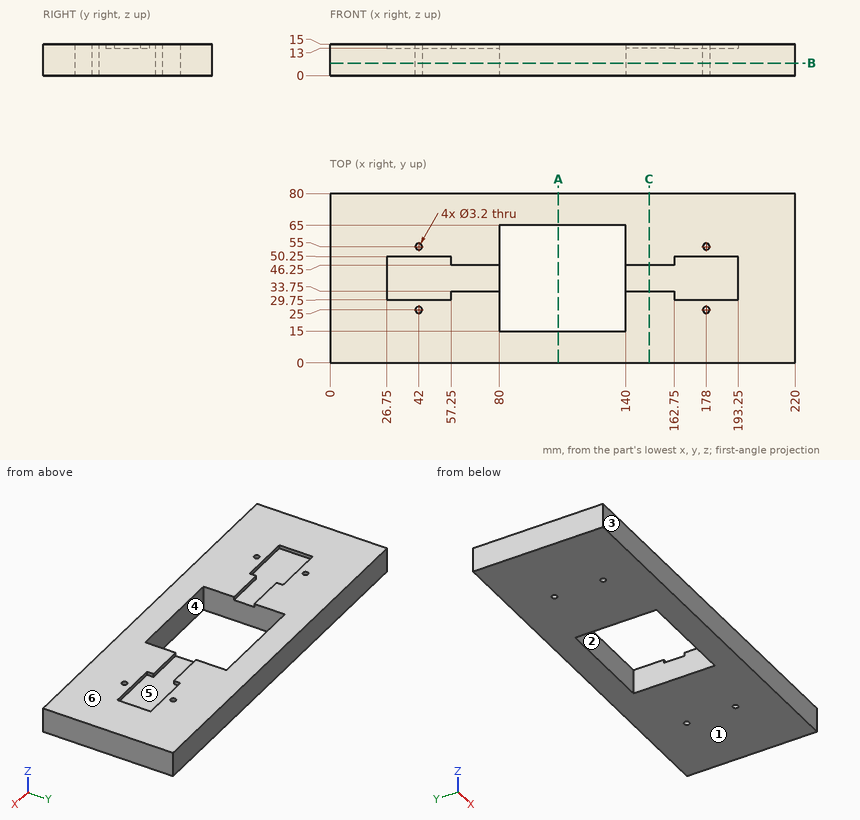
Part print with two shaded views. Sizes in mm from the minimum x, y, z corner. A direction names the side the tool comes from. Coordinates: 2 decimals unless noted, no trailing zeros. Write each loop counter-clockwise with the first axis right and the second up, starting at its lowest first coordinate (ties: lowest second). Pieces come first, ordered by that corner, then holes. Notation, with made-up numbers: M -29,-35.75 L 24,-35.75 A36 ccw 24,3.25 Z; hole C 45.25,30.25 d9. An arc over 180 degrees is marked long. Return JSON: item names as keys, results as strings.
Item 1: Which spindle directions (+Z, -Z, +X, -X, +Y, -Y) get a long thin tool onto all of the face, cutting with end or side? Do the marked faces 1 and 2. Say none if no direction does.
Findings below:
{"face 1": "-Z, +X, -X, +Y, -Y", "face 2": "+Z, -Z"}
Item 2: Slice it at B-B, the plane z = 6. Write the cut outline in (x, y).
Findings below:
{"outline": "M 0,0 L 220,0 L 220,80 L 0,80 Z; hole C 42,25 d3.2; hole C 42,55 d3.2; hole M 80,15 L 140,15 L 140,65 L 80,65 Z; hole C 178,25 d3.2; hole C 178,55 d3.2"}
Item 3: Two-plate mould, pull along Y, no slides. Class the marked faces 3, 4, 5 and 6: +Y half, -Y half, draft (parallel to the pull), parting line (faces both ways), or undercut.
Findings below:
{"face 3": "-Y half", "face 4": "undercut", "face 5": "undercut", "face 6": "draft"}
Item 4: Drop a flat-ended pin along its axis: pin 1 Ø1.9 at (x, y) = (178, 25) entering from -Z. Give the stop position or say it passes through.
Findings below:
{"pin 1": "passes through"}
Item 5: Probe line 1 (Y direction, x = 178, z = 11.75); line 2 (X direction, y = 36, z = 3); line 3 (Y direction, x = 131, z = 9.5). List the from-to ranges inside material, lowest first. Write a range as from..to.
Findings below:
{"line 1": "y = 0..23.4, 26.6..53.4, 56.6..80", "line 2": "x = 0..80, 140..220", "line 3": "y = 0..15, 65..80"}
Item 6: Slice it at C-C, the plane x = 151. Write the cut outline in (y, z), and give its area (4 significant figures).
Findings below:
{"outline": "M 0,0 L 80,0 L 80,15 L 46.25,15 L 46.25,13 L 33.75,13 L 33.75,15 L 0,15 Z", "area": "1,175 mm2"}
Item 7: Slice it at A-A, the plane x = 108. Write the cut outline in (y, z).
Findings below:
{"outline": "M 0,0 L 15,0 L 15,15 L 0,15 Z; M 65,0 L 80,0 L 80,15 L 65,15 Z"}
